Could you check a few things on this model? Use its own coordinates, in mm. A direction names the side the tool comes from. Coordinates: 2 decimals unless noted, no trailing zeros. Write each loop counter-clockwise with the first axis right and the second up, starting at its lowest first coordinate (ties: lowest second). Pieces come first, ordered by that corner, then holes.
```python
from build123d import *

# Parameters (mm, degrees)
EXTRUDE17_DEPTH = 1.6129
SKETCH19_R      = 3.6195
EXTRUDE19_DEPTH = 4.2291
SKETCH20_R      = 0.46355
SKETCH20_R_2    = 1.27
EXTRUDE20_DEPTH = 18.050548166
SKETCH21_R      = 2.44475
EXTRUDE21_DEPTH = 1.1557
SKETCH22_R      = 2.286
EXTRUDE22_DEPTH = 2.3368
SKETCH23_R      = 2.159
EXTRUDE23_DEPTH = 0.2032
SKETCH24_R      = 1.651
EXTRUDE24_DEPTH = 0.762
EXTRUDE25_DEPTH = 0.508
FILLET1_R       = 0.508


with BuildPart() as part:
    # Sketch18 → Extrude17 (new body)
    with BuildSketch(Plane(origin=(0, 0, 0), x_dir=(1, 0, 0), z_dir=(0, 1, 0))):
        with BuildLine():
            Line((-14.34305969, 1.923991942), (-2.13741415, 2.921))
            ThreePointArc((-2.13741415, 2.921), (3.6195, 0), (-2.13741415, -2.921))
            Line((-2.13741415, -2.921), (-14.34305969, -1.923991942))
            ThreePointArc((-14.34305969, -1.923991942), (-16.1163, 0), (-14.34305969, 1.923991942))
        make_face()
    extrude(amount=EXTRUDE17_DEPTH)

    # Sketch19 → Extrude19 (add)
    with BuildSketch(Plane(origin=(0, 1.6129, 0), x_dir=(1, 0, 0), z_dir=(0, 1, 0))):
        with Locations(Location((0, 0, 0), (0, 0, 126.194447475))):
            Circle(SKETCH19_R)
    extrude(amount=-EXTRUDE19_DEPTH)

    # Sketch20 → Extrude20 (cut, through all)
    with BuildSketch(Plane(origin=(0, 1.6129, 0), x_dir=(1, 0, 0), z_dir=(0, 1, 0))):
        with Locations(Location((-14.1859, 0, 0), (0, 0, 270))):
            Circle(SKETCH20_R)
        with Locations(Location((0, 0, 0), (0, 0, 270))):
            Circle(SKETCH20_R_2)
        with Locations(Location((-4.6609, 0, 0), (0, 0, 270))):
            Circle(SKETCH20_R)
        with Locations(Location((-6.5659, 0, 0), (0, 0, 270))):
            Circle(SKETCH20_R)
        with Locations(Location((-8.4709, 0, 0), (0, 0, 270))):
            Circle(SKETCH20_R)
        with Locations(Location((-10.3759, 0, 0), (0, 0, 270))):
            Circle(SKETCH20_R)
        with Locations(Location((-12.2809, 0, 0), (0, 0, 270))):
            Circle(SKETCH20_R)
    extrude(amount=-EXTRUDE20_DEPTH, mode=Mode.SUBTRACT)

    # Sketch21 → Extrude21 (cut)
    with BuildSketch(Plane(origin=(0, 1.6129, 0), x_dir=(1, 0, 0), z_dir=(0, 1, 0))):
        with Locations(Location((0, 0, 0), (0, 0, 270))):
            Circle(SKETCH21_R)
    extrude(amount=-EXTRUDE21_DEPTH, mode=Mode.SUBTRACT)

    # Sketch22 → Extrude22 (cut)
    with BuildSketch(Plane.XZ.offset(2.6162)):
        with Locations(Location((0, 0, 0), (0, 0, 270))):
            Circle(SKETCH22_R)
    extrude(amount=-EXTRUDE22_DEPTH, mode=Mode.SUBTRACT)



with BuildPart() as body_2:
    # Sketch23 → Extrude23 (new body)
    with BuildSketch(Plane(origin=(0, 0.4572, 0), x_dir=(1, 0, 0), z_dir=(0, 1, 0))):
        with Locations(Location((0, 0, 0), (0, 0, 270))):
            Circle(SKETCH23_R)
    extrude(amount=EXTRUDE23_DEPTH)


with BuildPart() as part_1:
    add(part.part)

    add(body_2.part)  # Extrude24 merges body 2
    # Sketch24 → Extrude24 (add)
    with BuildSketch(Plane(origin=(0, 0.6604, 0), x_dir=(1, 0, 0), z_dir=(0, 1, 0))):
        with Locations(Location((0, 0, 0), (0, 0, 90))):
            Circle(SKETCH24_R)
    extrude(amount=EXTRUDE24_DEPTH)

    # Sketch25 → Extrude25 (cut)
    with BuildSketch(Plane(origin=(0, 1.4224, 0), x_dir=(1, 0, 0), z_dir=(0, 1, 0))):
        Polygon((0.254, -1.016), (-0.254, -1.016), (-0.254, -0.254), (-1.016, -0.254), (-1.016, 0.254), (-0.254, 0.254), (-0.254, 1.016), (0.254, 1.016), (0.254, 0.254), (1.016, 0.254), (1.016, -0.254), (0.254, -0.254), align=None)
    extrude(amount=-EXTRUDE25_DEPTH, mode=Mode.SUBTRACT)

    # Fillet1
    fillet1_edges = [part_1.edges().sort_by_distance(p)[0] for p in [
        (0, 1.4224, 1.651),
    ]]
    fillet(fillet1_edges, radius=FILLET1_R)


solid = part_1.part
```
1. I want a section at D-D on x = -9.5. Please give me the cut outline in (y, z), plus the area to 3 significant figures.
Verdict:
outline: (0, -2.32) - (1.61, -2.32) - (1.61, 2.32) - (0, 2.32) - close
area: 7.48 mm2
2. I want a section at B-B on z = 0. Give the number of separate pieces and of enclosed holes in the cut face, plus the area to 3 significant figures.
Verdict:
separate pieces: 7
enclosed holes: 0
area: 25.8 mm2
3. On a 3-axis mill with a long thin cutter (end or side, diameter ignored), from which of +Z, -Z, +X, -X, +Y, -Y can I reach the whole of each face in a straight line? I mean faces 4 (the face through (-0.8, -2.616, -2.4)), 5 (the face through (-1.5, -0.279, 0)), 6 (the face through (-2, 0.66, 0)). Say none if no direction works.
Verdict:
face 4: +Z, -Z, +X, -X, -Y
face 5: -Y
face 6: +Y
4. If we mould it in two halves opening along X, with no side actions, what happens to faces 1 (the face through (-6, 1.613, 1)), 2 (the face through (-4.2, 0.82, -0.06)), 3 (the face through (-16.116, 0.795, 0.04))? For each: pulls with the +X half, pulls with the -X half, needs draft (parallel to the pull), parting line crosses it, or undercut.
Verdict:
face 1: needs draft
face 2: undercut
face 3: pulls with the -X half
5. For pin 1 (0.6 mm diameter, centred on x = 0, z = -0.5, fed in from +Y); pin 2 (2 mm diameter, centred on x = -12.5, y = 0, fed in from +Z); pin 3 (3 mm diameter, centred on x = 0.5, z = 0.5, fed in from -Y), each with a flat end and sliding along its axis, tell me the tip position at first contact or that it passes through.
Verdict:
pin 1: stops at y = 1.42
pin 2: stops at z = 2.16
pin 3: stops at y = -0.28
6. Please list where these lines run through material, in increasing order: line 1 along X through (y, z) = (-0.1, 0); line 2 along X through (y, z) = (-0.55, 0); line 3 along Y through (x, z) = (-8, 0.5).
Verdict:
line 1: x = -3.62 to -1.27, 1.27 to 3.62
line 2: x = -3.62 to -2.29, 2.29 to 3.62
line 3: y = 0 to 1.61
7. I want a section at C-C on y = -0.55. Please give me the cut outline in (x, z), plus the area to 3 significant figures.
Verdict:
outline: circle Ø7.24 at (0, 0); hole circle Ø4.57 at (0, 0)
area: 24.7 mm2
